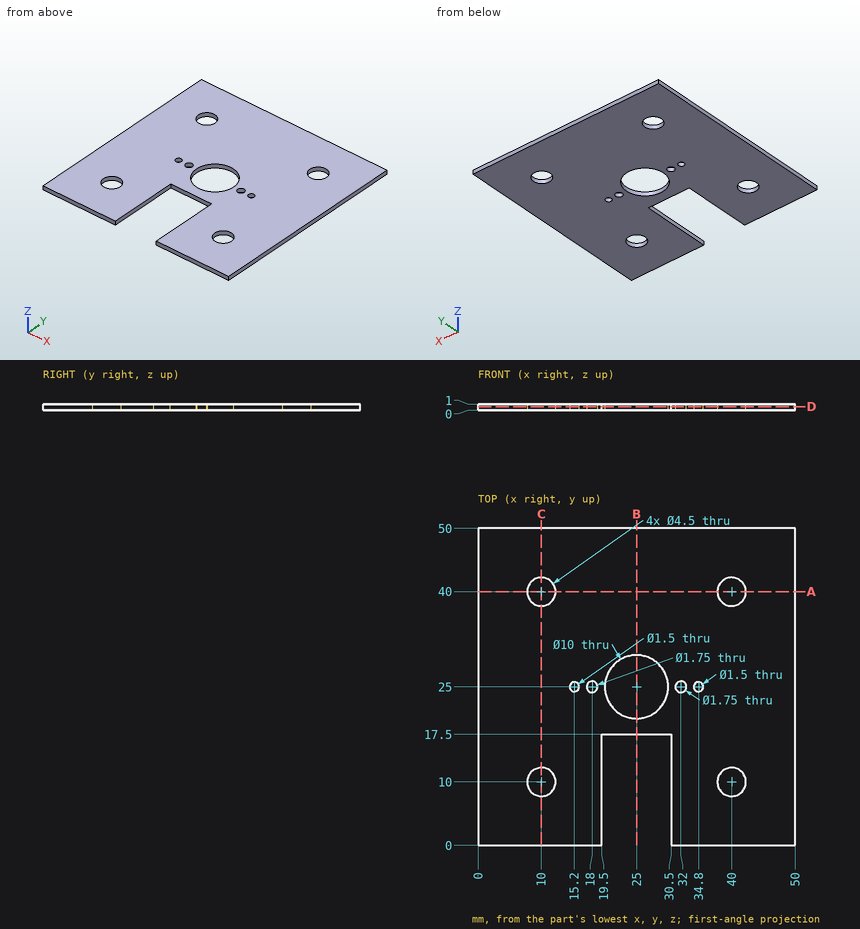
Here's the drawing with two shaded views (mm, measured from the low corner). I have some questions. Give positions to 0.01 mm unless a question says otherwise; leave off trailing zeros. Write each loop counter-clockwise with the first axis right and the second up, starting at its lowest first coordinate (ties: lowest second). Pieces come first, ordered by that corner, then holes. Notation, with made-up numbers: (23.25, -21.75) -> (42.25, -21.75) arc R18 ccw to (42.25, 4.25) -> close; hole circle Ø3 at (18, -27.75). An arc over 180 degrees is marked (long way). Answer as a JSON object with one key per item and string values. Group by question number.
Item 1: Suppose I cut it at B-B (x = 25). Please give me the cut outline in (y, z), plus the area to 3 significant figures.
Item 2: I'm going to push a flat-ended pin straight in: P1, Ø5, axis at x = 28.5, y = 14.5, coming from the +Z side. Where does the tip first touch, or does it pass through?
Item 3: Please list where these lines run through material, in increasing order: line 1 (Y direction, x = 10, z = 0.7); line 2 (Y direction, x = 34.8, z = 0.7); line 3 (X direction, y = 2, z = 0.3). Write a range as [from, to].
Item 4: Suppose I cut it at A-A (y = 40). Please give me the cut outline in (x, z).
Item 5: Suppose I cut it at D-D (z = 0.6). State how many separate pieces and enclosed holes the cut face has, plus the area to 3 significant figures.
Findings:
{
 "1": {"outline": "(17.5, 0) -> (20, 0) -> (20, 1) -> (17.5, 1) -> close; (30, 0) -> (50, 0) -> (50, 1) -> (30, 1) -> close", "area": "22.5 mm²"},
 "2": {"P1": "stops at z = 1"},
 "3": {"line 1": "y = [0, 7.75], [12.25, 37.75], [42.25, 50]", "line 2": "y = [0, 24.25], [25.75, 50]", "line 3": "x = [0, 19.5], [30.5, 50]"},
 "4": {"outline": "(0, 0) -> (7.75, 0) -> (7.75, 1) -> (0, 1) -> close; (12.25, 0) -> (37.75, 0) -> (37.75, 1) -> (12.25, 1) -> close; (42.25, 0) -> (50, 0) -> (50, 1) -> (42.25, 1) -> close"},
 "5": {"separate pieces": "1", "enclosed holes": "9", "area": "2,160 mm²"}
}
